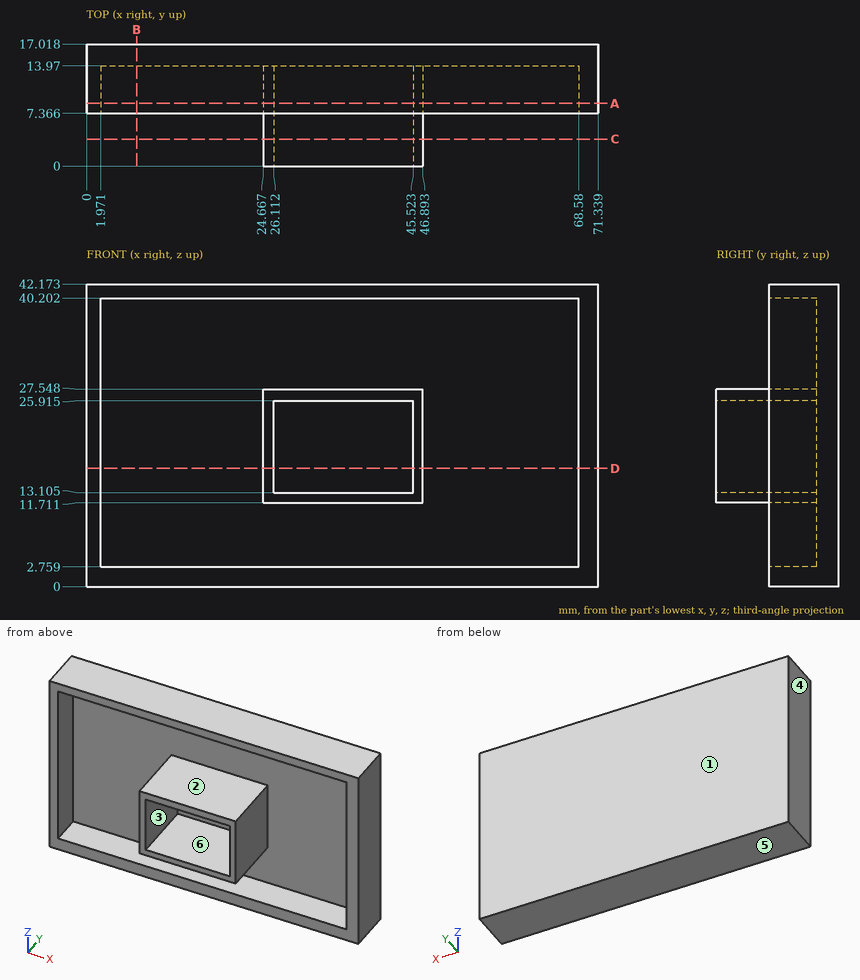
Geometry: see drawing. Coordinates: mm, zero at the bounding-box minimum. A direction names the side the tool comes from. Round coordinates to 2 decimals unless told otherwise and drop trailing zeros. Order: outer loops, then holes, each group sorted by start corner. A loop starts at its lowest first (then second) coordinate and runs counter-clockwise, first axis right, second up. Notation, with made-up numbers: (35.5, -11.5) -> (85.5, -11.5) arc R6 cw to (85.5, -6.5) -> close; hole circle Ø11 at (12.5, 1.5). An arc over 180 degrees is marked (long way). Answer as CSV lines item,"result".
Item 1: Section A-A, the plane y = 8.75. Return loops of the section in (x, z) (1 decimal).
A:
outline,"(0, 0) -> (71.3, 0) -> (71.3, 42.2) -> (0, 42.2) -> close; (24.7, 11.7) -> (46.9, 11.7) -> (46.9, 27.5) -> (24.7, 27.5) -> close; hole (2, 2.8) -> (68.6, 2.8) -> (68.6, 40.2) -> (2, 40.2) -> close; hole (26.1, 13.1) -> (45.5, 13.1) -> (45.5, 25.9) -> (26.1, 25.9) -> close"
Item 2: Pin query (flat end, axial travel): pin 1 Ø1.5 at (x, z) = (56.5, 7) entering from -Y; pin 2 Ø12 at (x, z) = (14.5, 4.5) entering from -Y. Return the tip coordinate at first contact, or that it passes through.
A:
pin 1,"y = 13.97"
pin 2,"y = 7.37"
Item 3: Section C-C, the plane y = 3.75. Return loops of the section in (x, z) (1 decimal).
A:
outline,"(24.7, 11.7) -> (46.9, 11.7) -> (46.9, 27.5) -> (24.7, 27.5) -> close; hole (26.1, 13.1) -> (45.5, 13.1) -> (45.5, 25.9) -> (26.1, 25.9) -> close"
Item 4: Reachability of the marked faces 1 and 2 from +Z, -Z, +X, -X, +Y, -Y: full face, straight path, thin tool, end or side. Return the list, or none.
A:
face 1,"+Z, -Z, +X, -X, +Y"
face 2,"-Y"
Item 5: Section D-D, the plane z = 16.5. Return loops of the section in (x, y).
A:
outline,"(0, 7.37) -> (1.97, 7.37) -> (1.97, 13.97) -> (24.67, 13.97) -> (24.67, 0) -> (26.11, 0) -> (26.11, 13.97) -> (45.52, 13.97) -> (45.52, 0) -> (46.89, 0) -> (46.89, 13.97) -> (68.58, 13.97) -> (68.58, 7.37) -> (71.34, 7.37) -> (71.34, 17.02) -> (0, 17.02) -> close"
Item 6: Line query: L1, parallel to Z at x = 29.5, y = 13 (1 decimal); L2, parallel to X at y = 4, z = 14; L3, parallel to Z at x = 54, y = 11.25. Output: solid intervals per line, ascending.
A:
L1,"0 to 2.8, 11.7 to 13.1, 25.9 to 27.5, 40.2 to 42.2"
L2,"24.67 to 26.11, 45.52 to 46.89"
L3,"0 to 2.76, 40.2 to 42.17"
Item 7: Section B-B, the plane x = 7. Return loops of the section in (y, z).
A:
outline,"(7.37, 0) -> (17.02, 0) -> (17.02, 42.17) -> (7.37, 42.17) -> (7.37, 40.2) -> (13.97, 40.2) -> (13.97, 2.76) -> (7.37, 2.76) -> close"
Item 8: Pull-direction query (Z, two-part tool) for the marked faces 3, 4, 5 and 6; classes: pulls with the +Z half, pulls with the -Z half, needs draft (parallel to the pull), parting line crosses it, or undercut.
A:
face 3,"undercut"
face 4,"needs draft"
face 5,"pulls with the -Z half"
face 6,"undercut"
